Can you work these out from the model? Positions are in its coordinate system, mm. A direction names the side the tool comes from. Give positions to 0.01 mm unless a question says otherwise; leave off trailing zeros. Write each loop counter-clockwise with the first axis right and the second up, starting at its lowest first coordinate (ties: lowest second). Pieces come first, ordered by that corner, then holes.
```python
from build123d import *

# Parameters (mm, degrees)
BOSS_EXTRUDE1_DEPTH = 0.7
CHAMFER1_SIZE       = 1
CHAMFER2_SIZE       = 0.5


with BuildPart() as part:
    # Sketch1 → Boss-Extrude1 (new body)
    with BuildSketch(Plane(origin=(0, 0, 0), x_dir=(1, 0, 0), z_dir=(0, 1, 0))):
        Polygon((0.284238857, 0.048748246), (4.822239021, 1.752850979), (11.041039678, 1.752850979), (14.137088798, 2.915474508), (17.798659013, 2.915474508), (29.070766186, 15.087446012), (32.094208001, 13.244081421), (32.986673125, 2.05865414), (33.011493829, 2.05865414), (36.605140674, 8.306952125), (39.91645027, 5.441925055), (39.11764025, 2.453830764), (37.15585938, 1.781640495), (37.15585938, -1.684144002), (39.11764025, -2.356334271), (39.91645027, -5.344428562), (36.605140674, -8.209455633), (33.011493829, -1.961157647), (32.986673125, -1.961157647), (32.094208001, -13.146584929), (29.070766186, -14.98994952), (17.798659013, -2.817978016), (14.137088798, -2.817978016), (11.041039678, -1.655354487), (4.822239021, -1.655354487), align=None)
    extrude(amount=BOSS_EXTRUDE1_DEPTH)

    # Chamfer1
    # the kernel refuses this chamfer: 1 mm, written as the material it takes off along each edge
    with BuildSketch(Plane(origin=(2.250556033, 0.7, -1.752850979), x_dir=(0, -0.9996219169112968, -0.02749587661058627), z_dir=(1, 0, 0))) as chamfer1_piece_1_section:
        Polygon((CHAMFER1_SIZE * 0.999621916911, -CHAMFER1_SIZE * 0.0274958766106), (-CHAMFER1_SIZE * 0.0274958766106, -CHAMFER1_SIZE * 0.999621916911), (0, 0), align=None)
    chamfer1_piece_1 = extrude(amount=11.362166633, mode=Mode.PRIVATE)
    chamfer1_piece_1 = split(chamfer1_piece_1, bisect_by=Plane(origin=(6.727578787, 0.358780421, -0.133066883), z_dir=(-0.3515489139570331, 0, -0.9361695151497034)), keep=Keep.TOP, mode=Mode.PRIVATE)
    add(chamfer1_piece_1, mode=Mode.SUBTRACT)
    with BuildSketch(Plane(origin=(-2.123292359, 0.7, 0.855324115), x_dir=(-0.00966614556074823, -0.9996219169112968, -0.025740801475148727), z_dir=(0.9361695151497034, 0, -0.351548913957033)), Plane(origin=(7.229770237, 0.7, 2.559426848), x_dir=(-0.00966614556074825, -0.9996219169112968, 0.025740801475148775), z_dir=(-0.9361695151497034, 0, -0.351548913957033))) as chamfer1_piece_2:
        Polygon((CHAMFER1_SIZE * 0.999621916911, -CHAMFER1_SIZE * 0.0274958766106), (-CHAMFER1_SIZE * 0.0274958766106, -CHAMFER1_SIZE * 0.999621916911), (0, 0), align=None)
    extrude(amount=9.990778854, mode=Mode.SUBTRACT)
    with BuildSketch(Plane(origin=(13.612722666, 0.7, 1.655354487), x_dir=(0, -0.9996219169112968, 0.02749587661058627), z_dir=(-1, 0, 0))) as chamfer1_piece_3_section:
        Polygon((CHAMFER1_SIZE * 0.999621916911, -CHAMFER1_SIZE * 0.0274958766106), (-CHAMFER1_SIZE * 0.0274958766106, -CHAMFER1_SIZE * 0.999621916911), (0, 0), align=None)
    chamfer1_piece_3 = extrude(amount=11.362166633, mode=Mode.PRIVATE)
    chamfer1_piece_3 = split(chamfer1_piece_3, bisect_by=Plane(origin=(6.727578787, 0.358780421, 0.035570391), z_dir=(-0.3515489139570331, 0, 0.9361695151497034)), keep=Keep.TOP, mode=Mode.PRIVATE)
    add(chamfer1_piece_3, mode=Mode.SUBTRACT)

    # Chamfer2
    chamfer2_edges = [part.edges().sort_by_distance(p)[0] for p in [
        (23.4347126, 0.7, 8.903963768),
        (32.540440563, 0.7, 7.553871288),
        (39.51704526, 0.7, 3.850381417),
        (37.15585938, 0.7, -0.048748246),
        (39.51704526, 0.7, -3.947877909),
        (32.540440563, 0.7, -7.65136778),
        (23.4347126, 0.7, -9.00146026),
    ]]
    chamfer(chamfer2_edges, length=CHAMFER2_SIZE)


solid = part.part
```
1) Suppose I cut it at C-C on x = 20. Write out the boundary of the cut face in (y, z).
Values follow:
outline: (0, -5.29) - (0.2, -5.29) - (0.7, -4.56) - (0.7, 4.46) - (0.2, 5.2) - (0, 5.2) - close
2) Suppose I cut it at B-B on y = 0.5. Write out the boundary of the cut face in (x, z), plus the area to 3 significant figures.
Values follow:
outline: (2.56, -0.05) - (4.97, -0.95) - (8.91, -0.95) - (14.14, -2.92) - (18.21, -2.92) - (29.33, -14.93) - (31.78, -13.44) - (32.69, -2.06) - (33.01, -2.06) - (36.61, -8.31) - (39.66, -5.66) - (38.78, -2.34) - (36.86, -1.68) - (36.86, 1.58) - (38.78, 2.24) - (39.66, 5.56) - (36.61, 8.21) - (33.01, 1.96) - (32.69, 1.96) - (31.78, 13.34) - (29.33, 14.83) - (18.21, 2.82) - (14.14, 2.82) - (8.91, 0.86) - (4.97, 0.86) - close
area: 399 mm2
3) Suppose I cut it at D-D on z = 10.5. Write out the boundary of the cut face in (x, y).
Values follow:
outline: (24.91, 0) - (32.31, 0) - (32.31, 0.2) - (31.8, 0.7) - (25.59, 0.7) - (24.91, 0.2) - close
4) For faces 1 (the face through (32.287, 0.447, 7.634)), 2 (the face through (34.833, 0.345, 5.129)), 3 (the face through (32.27, 0.45, -7.89)), which set-ups out of +Z, -Z, +X, -X, +Y, -Y let a thin tool reach every point of the face, with its end or its side?
Values follow:
face 1: +Z, +Y
face 2: +Z, +Y, -Y
face 3: -Z, +Y
5) Please list where these lines run through material, in increasing order: L1, parallel to X at y = 0.3, z = -5; L2, parallel to X at y = 0.45, z = 4; L3, parallel to Z at x = 38, y = 0.65.
Values follow:
L1: x = 19.87 to 32.65, 34.7 to 39.69
L2: x = 19.23 to 32.57, 34.18 to 39.3
L3: z = -7.1 to -2.07, 1.97 to 7
6) Suppose I cut it at A-A on z = -3.5. Write out the boundary of the cut face in (x, y), plus the area to 3 significant figures.
Values follow:
outline: (18.34, 0) - (32.87, 0) - (32.87, 0.2) - (32.37, 0.7) - (19.02, 0.7) - (18.34, 0.2) - close; (33.84, 0) - (39.4, 0) - (39.4, 0.2) - (38.88, 0.7) - (33.84, 0.7) - close
area: 13.6 mm2
7) If we mould it in two halves opening along Z, with no side actions, what happens to faces 4 (the face through (34.783, 0.345, -5.139)), 5 (the face through (23.7, 0.4, 8.9)), 6 (the face through (37.87, 0.35, 1.93))? For each: +Z half, -Z half, draft (parallel to the pull), parting line (faces both ways), or undercut.
Values follow:
face 4: -Z half
face 5: +Z half
face 6: undercut
